Source: CAD feature listing. Evaluate the final solid. Frame: model axes, mm. A direction names the side the tool comes from. Give positions to 0.01 mm unless a question says otherwise; leave off trailing zeros. Write each loop counter-clockwise with the first axis right and the second up, starting at its lowest first coordinate (ties: lowest second). Pieces come first, ordered by that corner, then holes. Notation, with made-up numbers: (12, -3.75) -> (66, -3.75) arc R22 cw to (66, 5.25) -> close; hole circle Ø2 at (68.5, -20). An arc over 180 degrees is marked (long way). Use one line per item in the form item = value. Start each with the question number.
(1) Cut plane B-B, the plane z = -3. Output: boundary loops of the cut face in (x, y).
(2) Cut plane C-C, the plane y = 4.5. Output: boundary loops of the cut face in (x, z), and give its area (3 significant figures).
(3) Draft query along Z for faces 3 (the face through (3, 2, 0)), 4 (the face through (0, 2, -3)), 5 (the face through (2.19, 5.77, -1.45)). Return one class per face: pulls with the +Z half, pulls with the -Z half, needs draft (parallel to the pull), parting line crosses it, or undercut.
(4) Cut plane D-D, the plane x = 1. Output: boundary loops of the cut face in (y, z).
(5) Set-up query: faces 1 (the face through (3, 0, -3)), 2 (the face through (4.4, 4, -1.6)). Return all of +Z, -Z, +X, -X, +Y, -Y with unobstructed straight access to the full face (end or side cutting, diameter ignored); none if empty.
(6) Material intervals for line 1 along X through (y, z) = (4.75, -2.9); line 2 along Y through (x, z) = (0.9, -3.2); line 3 along X through (y, z) = (7, -3.9), sorted ascending. Write a range as from..to.
(7) Cut plane A-A, the plane x = 3. Output: boundary loops of the cut face in (y, z).
Autodesk Inventor part; units mm, degrees
ref_plane "YZ Plane" through (0, 0, 0) normal (1, 0, 0) x (0, 1, 0)
ref_plane "XZ Plane" through (0, 0, 0) normal (0, 1, 0) x (-1, 0, 0)
ref_plane "XY Plane" through (0, 0, 0) normal (0, 0, 1) x (1, 0, 0)
sketch "Sketch1" plane through (0, 0, 0) normal (0, 1, 0) x (-1, 0, 0)
  line L0 (0, 0) -> (-6, 0)
  line L1 (-6, 0) -> (-6, -6)
  line L2 (-6, -6) -> (0, -6)
  line L3 (0, -6) -> (0, 0)
  circle A0 centre (-3, -3) radius 1.75
  dimension "d9" = 6
  dimension "d10" = 6
  dimension "d13" = 3.5
extrude "Extrusion3" add sketch "Sketch1" along normal blind 4 contours L3 L2 L1 L0 | A0
extrude "Extrusion4" add sketch "Sketch1" along normal blind 3.6 from surface at 4 contours A0
properties part number "ESP32_C3_SM"
Geometry says:
q1.outline = (0, 0) -> (6, 0) -> (6, 4) -> (4.75, 4) -> (4.75, 7.6) -> (1.25, 7.6) -> (1.25, 4) -> (0, 4) -> close
q2.outline = circle Ø3.5 at (3, -3)
q2.area = 9.62 mm^2
q3.face_3 = pulls with the +Z half
q3.face_4 = needs draft
q3.face_5 = parting line crosses it
q4.outline = (0, -6) -> (4, -6) -> (4, 0) -> (0, 0) -> close
q5.face_1 = +Z, -Z, +X, -X, -Y
q5.face_2 = +Y
q6.line_1 = 1.25..4.75
q6.line_2 = 0..4
q6.line_3 = 1.5..4.5
q7.outline = (0, -6) -> (4, -6) -> (4, -4.75) -> (7.6, -4.75) -> (7.6, -1.25) -> (4, -1.25) -> (4, 0) -> (0, 0) -> close
